For this review, take the finished solid that the model builds, in its own axes (mm). A direction names the side the tool comes from. Round coordinates to 2 decimals unless told otherwise and drop trailing zeros. Write each loop counter-clockwise with the first axis right and the second up, starting at its lowest first coordinate (ties: lowest second). Pieces come first, ordered by that corner, then holes. Notation, with made-up numbers: M -23,26 L -8,26 A23 ccw -8,37 Z; hole C 18.5,41 d1. An arc over 180 degrees is marked long. Write each question's results on one line, items separated by ' | '. Start each with the question number.
```python
from build123d import *

# Parameters (mm, degrees)
F0_W     = 25.4
F0_H     = 25.4
F1_DEPTH = 25.4
F2_T     = -3.81
F3_R     = 5.08
F5_W     = 16.256
F5_H     = 16.256
F6_DEPTH = 1.27
F7_W     = 14.732
F7_H     = 14.732
F8_DEPTH = 2.54


with BuildPart() as f1:
    # F0 (on Front) → F1 (new body)
    with BuildSketch(Plane.XZ):
        with Locations((-33.946944, 33.299525)):
            Rectangle(F0_W, F0_H)
    extrude(amount=F1_DEPTH)

    # F2
    f2_openings = [f1.faces().sort_by_distance(p)[0] for p in [
        (-33.946944, -12.7, 45.999525),
    ]]
    offset(amount=F2_T, openings=f2_openings)

    # F3
    f3_edges = [f1.edges().sort_by_distance(p)[0] for p in [
        (-46.646944, 0, 33.299525),
        (-46.646944, -25.4, 33.299525),
        (-21.246944, -25.4, 33.299525),
        (-21.246944, 0, 33.299525),
    ]]
    fillet(f3_edges, radius=F3_R)

    # F5 (on face) → F6 (cut)
    with BuildSketch(Plane.XY.offset(24.409525)):
        with Locations((-33.946944, -12.7)):
            Rectangle(F5_W, F5_H)
    extrude(amount=-F6_DEPTH, mode=Mode.SUBTRACT)

    # F7 (on face) → F8 (cut)
    with BuildSketch(Plane.XY.offset(24.409525)):
        with Locations((-33.946944, -12.7)):
            Rectangle(F7_W, F7_H)
    extrude(amount=-F8_DEPTH, mode=Mode.SUBTRACT)


solid = f1.part
```
Item 1: We need section A-A on x = -27.25. State the section outline as (y, z) points, then the cut area to 3 significant figures.
Item 2: For probe 1 along Y at (x, z) = (-39.25, 23.5); probe 2 along X at (y, z) = (-16.75, 45); probe 3 along X at (y, z) = (-8.75, 22), list the stretches that pass through material, from the lowest coordinate up.
Item 3: For faces 1 (the flat face through (-34.1, -20.066, 22.5)), 2 (the cylindrical face through (-45.2, -1.53, 33.48)), list the 3-axis set-ups (+Z, -Z, +X, -X, +Y, -Y) from which the entire face can be reached by the end or side of a thin tool; tool diameter is ignored.
Item 4: We need section C-C on y = -14.5. State the section outline as (x, z) points, then the cut area to 3 significant figures.
Item 5: We need section D-D on y = -2.75. State the section outline as (x, z) points, then the cut area to 3 significant figures.
Item 6: Insertion check: P1, Ø9, axis at x = -32.5, y = -16, coming from the +Z side; P2, Ø7.5, axis at x = -33.5, y = -12, coming from the +Z side; P3, Ø2, axis at y = -22, z = 40, coming from the -X side. Each pin has a flat end and moves straight along its axis. Give the tip position at first contact, or say it passes through.
Item 7: We need section B-B on z = 37.25. State the section outline as (x, y) points.
Item 8: Mouldability with a two-part tool opening along Y and no side actions: class faces 3 (the flat face through (-21.247, -13, 33)), 4 (the cylindrical face through (-22.696, -1.528, 33.477)), 5 (the flat face through (-34.1, -5.334, 22.5)) as pulls with the +Y half, pulls with the -Y half, needs draft (parallel to the pull), parting line crosses it, or undercut.
Numbers:
1) outline: M -25.4,20.6 L 0,20.6 L 0,46 L -3.81,46 L -3.81,24.41 L -4.57,24.41 L -4.57,23.14 L -5.33,23.14 L -5.33,21.87 L -20.07,21.87 L -20.07,23.14 L -20.83,23.14 L -20.83,24.41 L -21.59,24.41 L -21.59,46 L -25.4,46 Z | area: 222 mm^2
2) probe 1: y = -25.4 to -20.83, -4.57 to 0 | probe 2: x = -46.65 to -42.84, -25.06 to -21.25 | probe 3: x = -46.65 to -41.31, -26.58 to -21.25
3) face 1: +Z | face 2: +Z, -Z, -X, +Y
4) outline: M -46.65,20.6 L -21.25,20.6 L -21.25,46 L -25.06,46 L -25.06,24.41 L -25.82,24.41 L -25.82,23.14 L -26.58,23.14 L -26.58,21.87 L -41.31,21.87 L -41.31,23.14 L -42.07,23.14 L -42.07,24.41 L -42.84,24.41 L -42.84,46 L -46.65,46 Z | area: 222 mm^2
5) outline: M -46.08,20.6 L -21.81,20.6 L -21.81,46 L -46.08,46 Z | area: 616 mm^2
6) P1: stops at z = 23.14 | P2: stops at z = 21.87 | P3: stops at x = -46.6
7) outline: M -46.65,-20.32 A5.08 ccw -41.57,-25.4 L -26.33,-25.4 A5.08 ccw -21.25,-20.32 L -21.25,-5.08 A5.08 ccw -26.33,0 L -41.57,0 A5.08 ccw -46.65,-5.08 Z; hole M -42.84,-21.59 L -25.06,-21.59 L -25.06,-3.81 L -42.84,-3.81 Z
8) face 3: needs draft | face 4: pulls with the +Y half | face 5: undercut
